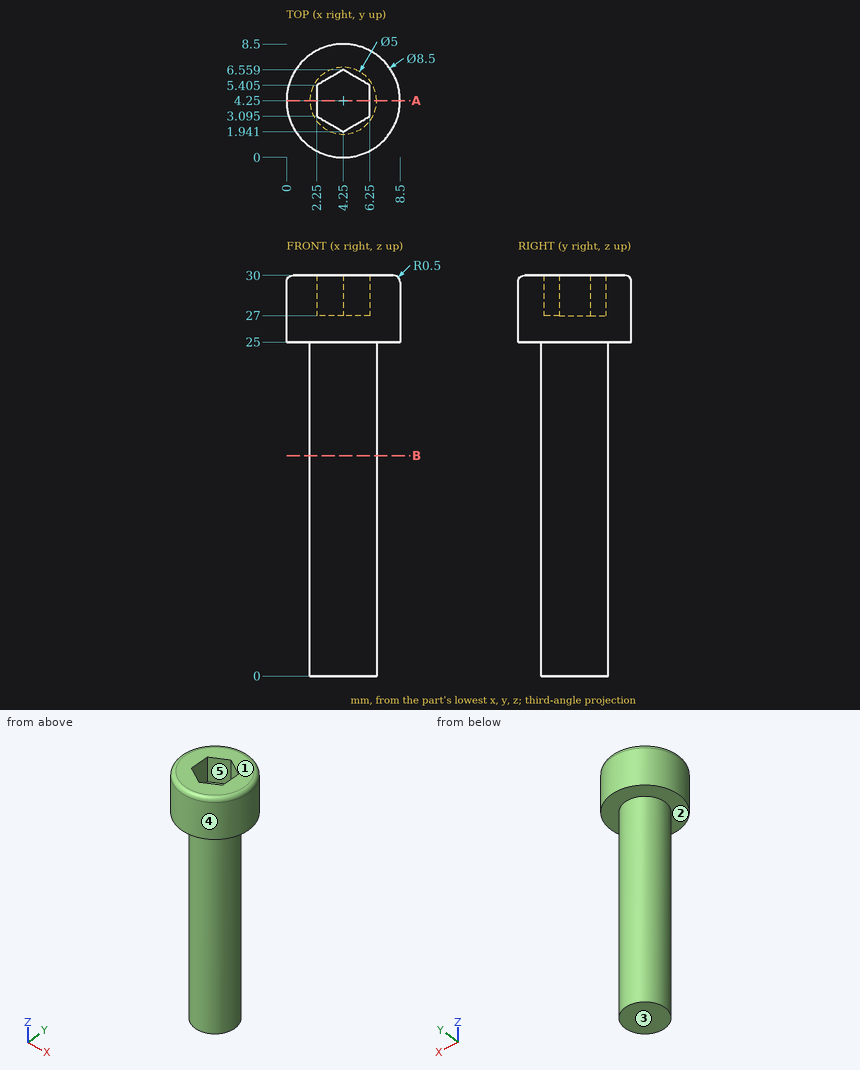
The drawing under review shows one solid part. Ordinate dimensions are in mm from its lowest x, y, z. A direction names the side the tool comes from. Round coordinates to 2 decimals unless told otherwise and drop trailing zeros. Write each loop counter-clockwise with the first axis right and the second up, starting at its lowest first coordinate (ties: lowest second). Pieces come first, ordered by that corner, then holes. Notation, with made-up numbers: (20, 81.5) - (71, 81.5) arc R18 cw to (71, 86.5) - close; hole circle Ø2 at (74.5, 8.5). An arc over 180 degrees is marked (long way). Put each result on its own line as item: value.
Q1. We need section B-B (z = 16.5). Give the boundary of the cut face in (x, y), and give its area (3 significant figures).
Solved:
outline: circle Ø5 at (4.25, 4.25)
area: 19.6 mm2
Q2. Machinability: for the marked faces 1 and 2, which of the approach directions +Z, -Z, +X, -X, +Y, -Y give a long, thin tool a straight path to every point of the face, cutting with its end or side? Answer none if there is none.
Solved:
face 1: +Z, +X, -X, +Y, -Y
face 2: -Z
Q3. We need section A-A (y = 4.25). Give the boundary of the cut face in (x, z), and give its area (3 significant figures).
Solved:
outline: (0, 25) - (1.75, 25) - (1.75, 0) - (6.75, 0) - (6.75, 25) - (8.5, 25) - (8.5, 29.5) arc R0.5 ccw to (8, 30) - (6.25, 30) - (6.25, 27) - (2.25, 27) - (2.25, 30) - (0.5, 30) arc R0.5 ccw to (0, 29.5) - close
area: 155 mm2
Q4. Wall thickness on probe 1 along Z at (x, y) = (3.5, 3.5); probe 2 along Z at (x, y) = (1.5, 6); probe 3 along Y at (x, z) = (3.5, 19.75) (1 decimal): over which ranges is each line inside the solid? List them lowest first.
Solved:
probe 1: z = 0 to 27
probe 2: z = 25 to 30
probe 3: y = 1.9 to 6.6
Q5. Mouldability with a two-part tool opening along Y and no side actions: class the marked faces 3, 4 and 5 as released by +Y, released by -Y, zero draft, split by the parting line, or undercut.
Solved:
face 3: zero draft
face 4: split by the parting line
face 5: undercut
Q6. Insertion check: pin 1 Ø1 at (x, y) = (3.5, 3.5) entering from +Z; pin 2 Ø1.5 at (x, z) = (7, 7.5) entering from -Y; pin 3 Ø3 at (x, z) = (3, 21.5) entering from -Y. Each pin has a flat end and moves straight along its axis. Give the tip position at first contact, or say it passes through.
Solved:
pin 1: stops at z = 27
pin 2: stops at y = 2.75
pin 3: stops at y = 1.75
